Source: CAD feature listing. Evaluate the final solid. Frame: model axes, mm. A direction names the side the tool comes from. Coordinates: 2 decimals unless noted, no trailing zeros. Write each loop counter-clockwise with the first axis right and the second up, starting at its lowest first coordinate (ties: lowest second). Pieces come first, ordered by that corner, then holes. Notation, with made-up numbers: (-30, -10) - (-16, -10) arc R34 ccw to (-16, 21) - close; hole circle Ø1 at (-32, 52). An arc over 180 degrees is marked (long way). One line per question, with ' | ' between items.
from build123d import *

# Parameters (mm, degrees)
SKETCH1_W           = 35
SKETCH1_H           = 46
BOSS_EXTRUDE1_DEPTH = 30
SKETCH2_W           = 31.5
SKETCH2_H           = 43
CUT_EXTRUDE1_DEPTH  = 28
FILLET1_R           = 2
FILLET2_R           = 1
SKETCH3_W           = 10
SKETCH3_H           = 28
CUT_EXTRUDE2_DEPTH  = 8


with BuildPart() as part:
    # Sketch1 → Boss-Extrude1 (new body)
    with BuildSketch(Plane(origin=(0, 0, 0), x_dir=(1, 0, 0), z_dir=(0, 1, 0))):
        Rectangle(SKETCH1_W, SKETCH1_H)
    extrude(amount=BOSS_EXTRUDE1_DEPTH)

    # Sketch2 → Cut-Extrude1 (cut)
    with BuildSketch(Plane(origin=(0, 30, 0), x_dir=(1, 0, 0), z_dir=(0, 1, 0))):
        Rectangle(SKETCH2_W, SKETCH2_H)
    extrude(amount=-CUT_EXTRUDE1_DEPTH, mode=Mode.SUBTRACT)

    # Fillet1
    fillet1_edges = [part.edges().sort_by_distance(p)[0] for p in [
        (17.5, 15, 23),
        (-17.5, 15, 23),
        (-17.5, 15, -23),
        (17.5, 15, -23),
    ]]
    fillet(fillet1_edges, radius=FILLET1_R)

    # Fillet2
    fillet2_edges = [part.edges().sort_by_distance(p)[0] for p in [
        (15.75, 16, -21.5),
        (15.75, 16, 21.5),
        (-15.75, 16, 21.5),
        (-15.75, 16, -21.5),
    ]]
    fillet(fillet2_edges, radius=FILLET2_R)

    # Sketch3 → Cut-Extrude2 (cut)
    with BuildSketch(Plane.XY.offset(23)):
        with Locations((0, 16)):
            Rectangle(SKETCH3_W, SKETCH3_H)
    extrude(amount=-CUT_EXTRUDE2_DEPTH, mode=Mode.SUBTRACT)


solid = part.part
Item 1: Pin query (flat end, axial travel): pin 1 Ø4 at (x, z) = (0, -4.5) entering from -Y; pin 2 Ø1.6 at (y, z) = (15.5, 22) entering from -X; pin 3 Ø1.6 at (y, z) = (17, 22.5) entering from +X; pin 4 Ø4 at (x, z) = (-0.5, -10.5) entering from +Y. Return the tip coordinate at first contact, or that it passes through.
Check sheet entries:
pin 1: y = 0 | pin 2: x = -17.49 | pin 3: x = 17.37 | pin 4: y = 2
Item 2: Cut plane C-C on z = -15.5. Return loops of the section in (x, y), and give its area (3 significant figures).
Check sheet entries:
outline: (-17.5, 0) - (17.5, 0) - (17.5, 30) - (15.75, 30) - (15.75, 2) - (-15.75, 2) - (-15.75, 30) - (-17.5, 30) - close | area: 168 mm²
Item 3: Access query for faces 1 (the face through (5, 16, 22)), 2 (the face through (0, 15, -23)), 3 (the face through (15.75, 16, 0)). Directions: +Z, -Z, +X, -X, +Y, -Y. A direction counts if a zero-diameter tool reaches every point of the face in a straight line with its end or side. Return the directions, or none.
Check sheet entries:
face 1: +Z, +Y | face 2: -Z, +X, -X, +Y, -Y | face 3: +Y
Item 4: Ray query, line 1 along X through (y, z) = (10.25, -6); line 2 along Z through (x, y) = (11, 23.25); line 3 along Y through (x, z) = (-6.5, -5). Return the intervals inside material, ascending. Write a range as [from, to].
Check sheet entries:
line 1: [-17.5, -15.75], [15.75, 17.5] | line 2: [-23, -21.5], [21.5, 23] | line 3: [0, 2]
Item 5: Cut plane A-A on y = 24. Return loops of the section in (x, z).
Check sheet entries:
outline: (-17.5, -21) arc R2 ccw to (-15.5, -23) - (15.5, -23) arc R2 ccw to (17.5, -21) - (17.5, 21) arc R2 ccw to (15.5, 23) - (5, 23) - (5, 21.5) - (14.75, 21.5) arc R1 cw to (15.75, 20.5) - (15.75, -20.5) arc R1 cw to (14.75, -21.5) - (-14.75, -21.5) arc R1 cw to (-15.75, -20.5) - (-15.75, 20.5) arc R1 cw to (-14.75, 21.5) - (-5, 21.5) - (-5, 23) - (-15.5, 23) arc R2 ccw to (-17.5, 21) - close
Item 6: Mould query, pull axis Z, two halves, no side actions, for faces 4 (the face through (-15.75, 16, 0)), 5 (the face through (-16.93, 15.21, -22.4)), 6 (the face through (16.9, 15.21, 22.43)). Classes: pulls with the +Z half, pulls with the -Z half, needs draft (parallel to the pull), parting line crosses it, or undercut.
Check sheet entries:
face 4: undercut | face 5: pulls with the -Z half | face 6: pulls with the +Z half
Item 7: Cut plane D-D on x = -11. Return loops of the section in (y, z).
Check sheet entries:
outline: (0, -23) - (30, -23) - (30, -21.5) - (2, -21.5) - (2, 21.5) - (30, 21.5) - (30, 23) - (0, 23) - close
Item 8: Cut plane B-B on x = -3. Return loops of the section in (y, z).
Check sheet entries:
outline: (0, -23) - (30, -23) - (30, -21.5) - (2, -21.5) - (2, 23) - (0, 23) - close
